from build123d import *

# Parameters (mm, degrees)
F1_DEPTH   = 152.4
F4_D       = 13.49248
F4_ON_F2_D = 13.49248


with BuildPart() as f1:
    # F0 (on Front) → F1 (new body, symmetric)
    with BuildSketch(Plane.XZ):
        with BuildLine():
            Line((-101.6, 1.905), (-101.6, 0))
            Line((-101.6, 0), (0, 0))
            Line((0, 0), (0, 101.6))
            Line((0, 101.6), (-1.905, 101.6))
            ThreePointArc((-1.905, 101.6), (-5.0480896424, 100.2980896424), (-6.35, 97.155))
            Line((-6.35, 97.155), (-6.35, 19.05))
            ThreePointArc((-6.35, 19.05), (-10.0697438789, 10.0697438789), (-19.05, 6.35))
            Line((-19.05, 6.35), (-97.155, 6.35))
            ThreePointArc((-97.155, 6.35), (-100.2980896424, 5.0480896424), (-101.6, 1.905))
        make_face()
    extrude(amount=F1_DEPTH, both=True)

    # F4 (through all)
    with Locations(Plane.YZ):
        with Locations((-50.8, 50.8), (50.8, 50.8)):
            Hole(F4_D / 2)

    # F4 on F2 (through all)
    with Locations(Plane(origin=(0, 0, 0), x_dir=(1, 0, 0), z_dir=(0, 0, -1))):
        with Locations((-50.8, 50.8), (-50.8, -50.8)):
            Hole(F4_ON_F2_D / 2)


solid = f1.part
Read the model definition and answer for the solid it produces. Units are mm, in the model's axes. A direction names the side the tool comes from. Coordinates: 2 decimals unless noted, no trailing zeros. Loops run counter-clockwise (first coordinate to the right, second up) from the corner with the lowest first, then second, coordinate; pieces in that order, holes last.
Q1. The part is cut by section B-B on z = 50.8. Write down the section's boundary in (x, y).
Q2. The part is cut by section C-C on x = -50.8. Write down the section's boundary in (y, z).
Q3. Each of these flat-tipped pins is pushed along its axis until it touches: pin 1 Ø8 at (y, z) = (-50.8, 50.8) entering from -X; pin 2 Ø6 at (x, y) = (-66.5, -66.5) entering from +Z; pin 3 Ø5 at (y, z) = (113.5, 69) entering from -X. Where does it stop, or does it pass through?
Q4. The part is cut by section A-A on y = 50.8. Write down the section's boundary in (x, z) (3 decimals).
Q5. The part is cut by section D-D on y = 130.5. Write down the section's boundary in (x, z) (3 decimals), and give its area (3 significant figures).
Q6. Which of the six approach directions +Z, -Z, +X, -X, +Y, -Y give full straight-line access (tool end or side, diameter ignored) to faces 1 (the face through (-6.35, -2, 59)), 2 (the face through (-3.219, 44.365, 52.826))?
Q7. Consider probe 1 along Y at (x, z) = (-50, 2); probe 2 along Z at (x, y) = (-1.5, 50.8); probe 3 along X at (y, z) = (-50.8, 2.25). Determine where each line is inside the solid, lowest interval first.
Q8. The mould has two halves that part along X. Classify faces 3 (the face through (-45.83, 46.24, 3.22)), 4 (the face through (-9.97, -2.13, 10.17)), 5 (the face through (-52, -2, 0)): +X half, -X half, draft (parallel to the pull), parting line (faces both ways), or undercut.
Results below:
1. outline: (-6.35, -152.4) - (0, -152.4) - (0, -57.55) - (-6.35, -57.55) - close; (-6.35, -44.05) - (0, -44.05) - (0, 44.05) - (-6.35, 44.05) - close; (-6.35, 57.55) - (0, 57.55) - (0, 152.4) - (-6.35, 152.4) - close
2. outline: (-152.4, 0) - (-57.55, 0) - (-57.55, 6.35) - (-152.4, 6.35) - close; (-44.05, 0) - (44.05, 0) - (44.05, 6.35) - (-44.05, 6.35) - close; (57.55, 0) - (152.4, 0) - (152.4, 6.35) - (57.55, 6.35) - close
3. pin 1: passes through
3. pin 2: stops at z = 6.35
3. pin 3: stops at x = -6.35
4. outline: (-101.6, 0) - (-57.546, 0) - (-57.546, 6.35) - (-97.155, 6.35) arc R4.445 ccw to (-101.6, 1.905) - close; (-44.054, 0) - (0, 0) - (0, 44.054) - (-6.35, 44.054) - (-6.35, 19.05) arc R12.7 cw to (-19.05, 6.35) - (-44.054, 6.35) - close; (-6.35, 57.546) - (0, 57.546) - (0, 101.6) - (-1.905, 101.6) arc R4.445 ccw to (-6.35, 97.155) - close
5. outline: (-101.6, 0) - (0, 0) - (0, 101.6) - (-1.905, 101.6) arc R4.445 ccw to (-6.35, 97.155) - (-6.35, 19.05) arc R12.7 cw to (-19.05, 6.35) - (-97.155, 6.35) arc R4.445 ccw to (-101.6, 1.905) - close
5. area: 1,280 mm2
6. face 1: +Z, -X, +Y, -Y
6. face 2: +X, -X
7. probe 1: y = -152.4 to -57.5, -44.1 to 44.1, 57.5 to 152.4
7. probe 2: z = 0 to 44.05, 57.55 to 101.6
7. probe 3: x = -101.59 to -57.55, -44.05 to 0
8. face 3: undercut
8. face 4: -X half
8. face 5: draft
